Can you work these out from the model? Positions are in its coordinate system, mm. A direction names the side the tool comes from. Give positions to 0.01 mm unless a question says otherwise; leave off trailing zeros. Order: outer loops, then holes, each group sorted by start corner. A loop starts at its lowest first (then second) coordinate and runs counter-clockwise, first axis right, second up.
Item 1: I'm going to push flat-ended pins straight in: pin 1 Ø1 at (x, z) = (-11, 48) entering from -Y; pin 2 Ø4 at (x, z) = (-9.5, 32) entering from +Y; pin 3 Ø5 at (y, z) = (-3, 43) entering from -X; pin 4 Ø8 at (x, y) = (-0.5, -15) entering from -Z. Where does each tip first touch, or does it pass through?
Item 2: I want a section at B-B, the plane z = 11.5. Write out the boundary of the cut face in (x, y), then the cut area to 3 significant figures.
Item 3: If we mould it in two halves opening along X, with no side actions, what happens to faces 4 (the conical face through (-3.593, -16.182, 27.77)), 5 (the flat face through (-0.1, -21.2, 65)), 6 (the conical face through (-2.98, -13.42, 28.77))? For each: +X half, -X half, draft (parallel to the pull), parting line (faces both ways), or undercut.
Item 4: If I drill on line 1 along Y through (x, z) = (0, 9.75); line 2 along Y through (x, z) = (0, 61); line 3 along X through (y, z) = (0, 15), over which ranges is the centre line in solid material (lowest first)?
Item 5: Which directions (+Z, -Z, +X, -X, +Y, -Y) give clear straight access to the entire face, cutting with the end or side of a thin tool? Please do faces 1 (the cylindrical face through (-23.977, 1.055, 59.74)), 2 (the cylindrical face through (11.923, 3.755, 5.409)), 3 (the cylindrical face through (20.03, 6.31, 59.74)).
Item 6: I want a section at A-A, the plane z = 59. Write out the boundary of the cut face in (x, y), then the cut area to 3 significant figures.
```python
from build123d import *

# Parameters (mm, degrees)
F5_T     = -3
F4_R     = 10.5
F6_DEPTH = 65.001


with BuildPart() as f2:
    # F1 (on Front) → F2 (revolve)
    with BuildSketch(Plane.XZ):
        with BuildLine():
            Line((0, 65), (0, 0))
            Line((0, 0), (12.5, 0))
            Line((12.5, 0), (12.5, 10.6695285708))
            ThreePointArc((12.5, 10.6695285708), (12.9687621154, 16.169510351), (14.3615261282, 21.51083471))
            Line((14.3615261282, 21.51083471), (22.1384738718, 43.48916529))
            ThreePointArc((22.1384738718, 43.48916529), (23.5312378846, 48.830489649), (24, 54.3304714292))
            Line((24, 54.3304714292), (24, 65))
            Line((24, 65), (0, 65))
        make_face()
    revolve(axis=Axis((0, 0, 32.5), (0, 0, 1)))

    # F5
    f5_openings = [f2.faces().sort_by_distance(p)[0] for p in [
        (0, 0, 65),
    ]]
    offset(amount=F5_T, openings=f5_openings)

    # F4 (on face) → F6 (cut, through all)
    with BuildSketch(Plane(origin=(0, 0, 0), x_dir=(1, 0, 0), z_dir=(0, 0, -1))):
        Circle(F4_R)
    extrude(amount=-F6_DEPTH, mode=Mode.SUBTRACT)


solid = f2.part
```
Results list:
1. pin 1: stops at y = -20.91
1. pin 2: stops at y = 16.73
1. pin 3: stops at x = -22.63
1. pin 4: stops at z = 0
2. outline: circle Ø25.02 at (0, 0); hole circle Ø21 at (0, 0)
2. area: 145 mm2
3. face 4: parting line
3. face 5: draft
3. face 6: undercut
4. line 1: y = -12.5 to -10.5, 10.5 to 12.5
4. line 2: y = -24 to -21, 21 to 24
4. line 3: x = -12.79 to -10.5, 10.5 to 12.79
5. face 1: +Z, -Z
5. face 2: -Z
5. face 3: +Z
6. outline: circle Ø48 at (0, 0); hole circle Ø42 at (0, 0)
6. area: 424 mm2
